Solid Edge part; units mm, degrees
sketch "Sketch1" plane through (0, 0, 0) normal (0, -1, 0) x (1, 0, 0)
  line L0 (0, 0) -> (0, 200)
  line L1 (0, 200) -> (100, 200)
  line L2 (100, 200) -> (100, 0)
sketch "Sketch2" plane through (0, 0, 0) normal (0, 0, 1) x (1, 0, 0)
  circle A0 centre (0, 0) radius 10
sweep "SweptProtrusion_1" add profiles "Sketch2" path "Sketch1"
sketch "Sketch3" plane through (0, 0, 0) normal (0, 1, 0) x (-1, 0, 0)
  line L0 (-4, 55.88) -> (-4, 35.88)
  line L1 (-4, 35.88) -> (4, 35.88)
  line L2 (4, 35.88) -> (4, 55.88)
  line L3 (4, 55.88) -> (-4, 55.88)
extrude "ExtrudedProtrusion_1" add sketch "Sketch3" along normal blind 35
sketch "Sketch4" plane through (-4, 14.5826, 70) normal (-1, 0, 0) x (0, -1, 0)
  circle A0 centre (-13.4174, -24.12) radius 4
extrude "ExtrudedCutout_1" cut sketch "Sketch4" against normal blind 16.5198
mirror "Mirror1" about plane through (50, 0, 0) normal (-1, 0, 0) of "ExtrudedProtrusion_1", "ExtrudedCutout_1"
sketch "Sketch5" plane through (10, 0, 105) normal (1, 0, 0) x (0, 0, 1)
  circle A0 centre (-95, 0) radius 5
extrude "ExtrudedCutout_2" cut sketch "Sketch5" along normal mid plane 237.1494
properties material "Stainless steel"
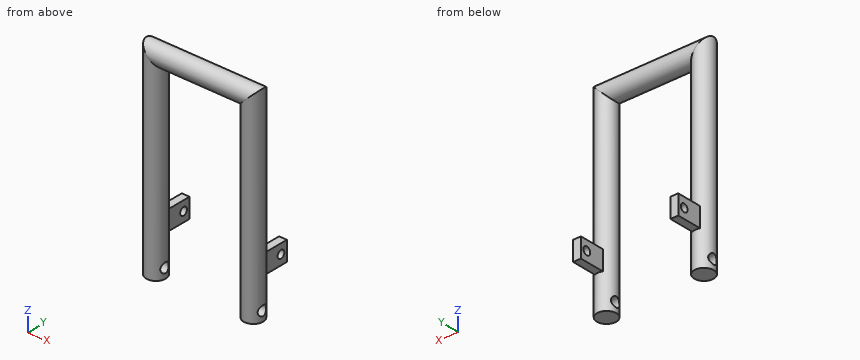
Design review of the part built by this model. Coordinates are the model's own, in mm. Coordinates: 2 decimals unless noted, no trailing zeros. Write each loop counter-clockwise with the first axis right and the second up, starting at its lowest first coordinate (ties: lowest second). Pieces come first, ordered by that corner, then holes.
1) Add section D-D (y = 15). Write out the cut boundary in (x, z), plus the area to 3 significant figures.
2) Add section B-B (x = 100). Write out the cut boundary in (y, z).
3) Add section A-A (y = 0). Write out the cut boundary in (x, z).
4) Insertion check: pin 1 (6 mm diameter, centred on y = 0, z = 10, fed in from +X); pin 2 (6 mm diameter, centred on y = 16, z = 53, fed in from -X); pin 3 (4 mm diameter, centred on x = -1, y = 16.5, fed in from +Z); pin 4 (6 mm diameter, centred on x = 97.5, y = 30, fed in from -Z). Each pin has a flat end and moves straight along its axis. Give the tip position at first contact, or say it passes through.
5) Add section C-C (z = 119). Write out the cut boundary in (x, y), plus the area to 3 significant figures.
6) To check wall thickness, follow L1, parallel to X at y = -0.5, z = 27; L2, parallel to Z at x = -2, y = 28; L3, parallel to Y at x = 100.25, z = 10. State the ranges of each line that lie inside material, in increasing order.
Check result:
1. outline: (-4, 35.88) - (4, 35.88) - (4, 55.88) - (-4, 55.88) - close; (96, 35.88) - (104, 35.88) - (104, 55.88) - (96, 55.88) - close
1. area: 320 mm2
2. outline: (-10, 0) - (10, 0) - (10, 35.88) - (35, 35.88) - (35, 55.88) - (10, 55.88) - (10, 200) arc R10 ccw to (-10, 200) - close; hole circle Ø10 at (0, 10); hole circle Ø8 at (28, 45.88)
3. outline: (-10, 0) - (10, 0) - (10, 5) - (-10, 5) - close; (-10, 15) - (10, 15) - (10, 190) - (90, 190) - (90, 15) - (110, 15) - (110, 210) - (-10, 210) - close; (90, 0) - (110, 0) - (110, 5) - (90, 5) - close
4. pin 1: passes through
4. pin 2: stops at x = -4
4. pin 3: stops at z = 55.88
4. pin 4: stops at z = 35.88
5. outline: circle Ø20 at (0, 0); circle Ø20 at (100, 0)
5. area: 628 mm2
6. L1: x = -9.99 to 9.99, 90.01 to 109.99
6. L2: z = 35.88 to 41.88, 49.88 to 55.88
6. L3: y = -10 to -5, 5 to 10
